Check sheet for the modelled part. Datum: model origin and axes. Units: mm. A direction names the side the tool comes from. Round coordinates to 2 decimals unless told otherwise and drop trailing zeros. Write each loop counter-clockwise with the first axis right and the second up, starting at its lowest first coordinate (ties: lowest second). Pieces come first, ordered by that corner, then holes.
Item 1: Section check B-B, the plane z = -2.25. State how many separate pieces and enclosed holes the cut face has, plus the area to 3 significant figures.
Item 2: Material ranges on line 1 along X through (y, z) = (0.5, -4.25); line 2 along X through (y, z) = (-3.5, -1.5); line 3 along X through (y, z) = (-2, -4.75), recorded low to high.
Item 3: Section check A-A, the plane z = -5. Record the cut outline in (x, y).
Item 4: Set-up check for faces 3 (the flat face through (-2.9, 0, -3)), 4 (the flat face through (-0.1, 2.2, -6)), 5 (the conical face through (-3.793, 0.076, -2.958)): record each of +Z, -Z, +X, -X, +Y, -Y from which the full face is reachable in a straight line by a thin tool's end or side.
Item 5: Depth check by flat-ended pin: pin 1 (0.5 mm diameter, centred on x = 2.5, z = -3.5, fed in from +Y); pin 2 (0.5 mm diameter, centred on y = 2, z = -3, fed in from +X); pin 3 (1 mm diameter, centred on y = -3, z = -2.5, fed in from -X). Enter the tip coordinate at first touch or a pass-through.
Item 6: Release check for a two-part mould opening along X. For faces 1 (the flat face through (-1, 2.4, -3)), 2 (the flat face through (-2.4, 0, -6)) record: pulls with the +X half, pulls with the -X half, needs draft (parallel to the pull), parting line crosses it, or undercut.
from build123d import *

# Parameters (mm, degrees)
SKETCH001_W  = 1
SKETCH001_H  = 3.8
PAD_DEPTH    = 6
PAD001_DEPTH = 4.2


with BuildPart() as part:
    # Sketch → Revolution (revolve)
    with BuildSketch(Plane.XZ):
        Polygon((0, 1), (4.85, 1), (4.75, -6), (3.75, -6), (3.835714, 0), (0, 0), align=None)
    revolve(axis=Axis((0, 0, 0), (0, 0, 1)))

    # Sketch001 → Pad (new body)
    with BuildSketch(Plane.XY):
        Polygon((-1, -1.9), (-1, -2.9), (-0.5, -2.9), (-0.5, -4.35), (0.5, -4.35), (0.5, -2.9), (1, -2.9), (1, -1.9), align=None)
        Polygon((-1, 2.9), (-1, 1.9), (1, 1.9), (1, 2.9), (0.5, 2.9), (0.5, 4.35), (-0.5, 4.35), (-0.5, 2.9), align=None)
        with Locations((2.4, 0)):
            Rectangle(SKETCH001_W, SKETCH001_H)
        with Locations((-2.4, 0)):
            Rectangle(SKETCH001_W, SKETCH001_H)
    extrude(amount=-PAD_DEPTH)

    # Sketch002 → Pad001 (join)
    with BuildSketch(Plane.XY):
        Polygon((-0.5, 2.5), (-0.5, 0.5), (-2.5, 0.5), (-2.5, -0.5), (-0.5, -0.5), (-0.5, -2.5), (0.5, -2.5), (0.5, -0.5), (2.5, -0.5), (2.5, 0.5), (0.5, 0.5), (0.5, 2.5), align=None)
    extrude(amount=-PAD001_DEPTH)


solid = part.part
Values found:
1. separate pieces: 1
1. enclosed holes: 2
1. area: 47.0 mm2
2. line 1: x = -4.75 to -3.74, -2.9 to -1.9, 1.9 to 2.9, 3.74 to 4.75
2. line 2: x = -3.31 to -1.52, -0.5 to 0.5, 1.52 to 3.31
2. line 3: x = -4.33 to -3.19, -1 to 1, 3.19 to 4.33
3. outline: circle Ø9.53 at (0, 0); (-2.9, -1.9) - (-1.9, -1.9) - (-1.9, 1.9) - (-2.9, 1.9) - close; (1.9, -1.9) - (2.9, -1.9) - (2.9, 1.9) - (1.9, 1.9) - close; hole (-1, -2.9) - (-1, -1.9) - (1, -1.9) - (1, -2.9) - (0.5, -2.9) - (0.5, -3.73) arc R3.76 ccw to (0.5, 3.73) - (0.5, 2.9) - (1, 2.9) - (1, 1.9) - (-1, 1.9) - (-1, 2.9) - (-0.5, 2.9) - (-0.5, 3.73) arc R3.76 ccw to (-0.5, -3.73) - (-0.5, -2.9) - close
4. face 3: -Z
4. face 4: -Z, +X, -X, +Y, -Y
4. face 5: none
5. pin 1: stops at y = 4.22
5. pin 2: stops at x = 4.46
5. pin 3: stops at x = -4.1
6. face 1: undercut
6. face 2: needs draft
